The listing builds one solid part. Answer for the finished solid, in the listing's coordinates (mm). Face numbers are marked on the shaded views. A direction names the side the tool comes from. Round coordinates to 2 decimals unless told otherwise and drop trailing zeros. Write each loop counter-clockwise with the first axis right and the second up, starting at its lowest first coordinate (ties: lowest second). Pieces come first, ordered by that corner, then holes. Notation, with made-up numbers: M -0.5,37 L 16.5,37 A21 cw 16.5,52 Z; hole C 29.5,-30.5 d10. An arc over 180 degrees is marked long. Answer as CSV lines item,"result". Start each with the question number.
from build123d import *

# Parameters (mm, degrees)
SKETCH1_R           = 2.75
BOSS_EXTRUDE1_DEPTH = 6
BODY_START          = 3
SKETCH2_R           = 2.75
BODY_HOLE_DEPTH     = 3
CUT_EXTRUDE2_DEPTH  = 23.226110771
CUT_REVOLVE1_ANGLE  = 180
SKETCH7_R           = 0.8
SCREW_HOLES_DEPTH   = 22.656407828
SKETCH9_R           = 1.25
SCREW_HEADS_DEPTH   = 4


with BuildPart() as part:
    # Sketch1 → Boss-Extrude1 (new body)
    with BuildSketch(Plane.XY):
        with BuildLine():
            Line((17, -12), (17, 12))
            Line((17, 12), (5, 12))
            ThreePointArc((5, 12), (-13, 0), (5, -12))
            Line((5, -12), (17, -12))
        make_face()
        Circle(SKETCH1_R, mode=Mode.SUBTRACT)
    extrude(amount=BOSS_EXTRUDE1_DEPTH)

    # Sketch2 → Body Hole (cut)
    with BuildSketch(Plane.XY.offset(BODY_START)):
        with BuildLine():
            ThreePointArc((5, 12), (-13, 0), (5, -12))
            Line((5, -12), (13, -12))
            Line((13, -12), (13, -4.25))
            Line((13, -4.25), (17, -4.25))
            Line((17, -4.25), (17, 4.25))
            Line((17, 4.25), (13, 4.25))
            Line((13, 4.25), (13, 12))
            Line((13, 12), (5, 12))
        make_face()
        Circle(SKETCH2_R, mode=Mode.SUBTRACT)
    extrude(amount=BODY_HOLE_DEPTH, mode=Mode.SUBTRACT)

    # Sketch3 → Cut-Extrude2 (cut, through all)
    with BuildSketch(Plane(origin=(0, 0, 0), x_dir=(0, 0, -1), z_dir=(1, 0, 0))):
        with BuildLine():
            Line((2, 15), (-13, 15))
            ThreePointArc((-13, 15), (-2.393398282, 10.606601718), (2, 0))
            Line((2, 0), (2, 15))
        make_face()
        with BuildLine():
            Line((2, -15), (2, 0))
            ThreePointArc((2, 0), (-2.393398282, -10.606601718), (-13, -15))
            Line((-13, -15), (2, -15))
        make_face()
    extrude(amount=CUT_EXTRUDE2_DEPTH, mode=Mode.SUBTRACT)

    # Sketch6 → Cut-Revolve1 (revolve, cut)
    with BuildSketch(Plane(origin=(0, 0, 0), x_dir=(0, 0, -1), z_dir=(1, 0, 0))):
        with BuildLine():
            Line((1, 15), (-13, 15))
            ThreePointArc((-13, 15), (-4.508164866, 12.36481848), (1, 5.385164807))
            Line((1, 5.385164807), (2, 5.385164807))
            Line((2, 5.385164807), (2, 15))
            Line((2, 15), (1, 15))
        make_face()
    revolve(axis=Axis((0, 0, 0), (0, 0, 1)), revolution_arc=CUT_REVOLVE1_ANGLE, mode=Mode.SUBTRACT)

    # Sketch7 → Screw Holes (cut, through all)
    with BuildSketch(Plane.XY):
        with Locations(Location((15, 10, 0), (0, 0, 180))):
            Circle(SKETCH7_R)
        with Locations(Location((15, -10, 0), (0, 0, 180))):
            Circle(SKETCH7_R)
    extrude(amount=SCREW_HOLES_DEPTH, mode=Mode.SUBTRACT)

    # Sketch9 → Screw Heads (cut)
    with BuildSketch(Plane.XY):
        with Locations(Location((15, 10, 0), (0, 0, 180))):
            Circle(SKETCH9_R)
    extrude(amount=SCREW_HEADS_DEPTH, mode=Mode.SUBTRACT)


solid = part.part
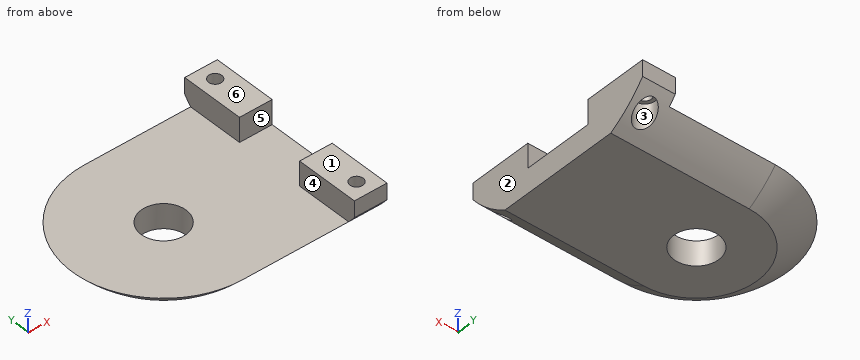
Q1. For the marked faces 4, 5 and 6, determine the directions among +Z, -Z, +X, -X, +Y, -Y from which every point of the face is accessible in a straight line to the end or side of a thin tool.
Q2. Straight lines are drawn through the part: L1, parallel to Y at x = 15, z = 5.05; L2, parallel to X at y = -10, z = 4.8; L3, parallel to Z at x = 14.5, y = 2. For each, find the intervals that lie inside material, in ascending order.
Q3. Find section B-B (y = 0). Determine the outline of the cut face in (x, z), plus the area to 3 significant figures.
Q4. Find section D-D (x = -2). Determine the outline of the cut face in (y, z).
Q5. Each of these flat-tipped pins is pushed along its axis until it touches: P1, Ø4, axis at x = -8, y = -2, coming from the +Z side; P2, Ø3, axis at x = 15, y = 10.5, coming from the -Z side; P3, Ø3.5, axis at x = 0, y = 0, coming from the -Z side; P4, Ø2, axis at y = 7, z = 1.5, coming from the -X side. Where does it stop, or does it pass through?
Q6. The mould has two halves that part along X. Classify the marked faces 1, 2 and 3: +X half, -X half, draft (parallel to the pull), parting line (faces both ways), or undercut.
Q7. Find section A-A (z = 5.25). Determine the outline of the cut face in (x, y).
Q8. Find section C-C (x = 15). Determine the outline of the cut face in (y, z), plus the area to 3 significant figures.
Reported:
1,face 4,"+Z, -X, +Y, -Y"
1,face 5,"+Z, +X, -X"
1,face 6,"+Z, +X, -X, +Y, -Y"
2,L1,"y = -12 to -10.8, -9.2 to -4.25, 4.25 to 9.2, 10.8 to 12"
2,L2,"x = 13 to 14.2, 15.8 to 17"
2,L3,"z = 0 to 3"
3,outline,"M -11.18,3 A15 ccw -7.48,0 L -2.75,0 L -2.75,3 Z; M 2.75,0 L 17,0 L 17,3 L 2.75,3 Z"
3,area,"63.1 mm2"
4,outline,"M -11,3 A14.87 ccw -7.21,0 L -1.89,0 L -1.89,3 Z; M 1.89,0 L 7.21,0 A14.87 ccw 11,3 L 1.89,3 Z"
5,P1,"stops at z = 3"
5,P2,"stops at z = 1.44"
5,P3,"passes through"
5,P4,"stops at x = -8.35"
6,face 1,"draft"
6,face 2,"+X half"
6,face 3,"undercut"
7,outline,"M 13,-12 L 17,-12 L 17,-4.25 L 13,-4.25 Z; M 13,4.25 L 17,4.25 L 17,12 L 13,12 Z; hole C 15,-10 d1.6; hole C 15,10 d1.6"
8,outline,"M -12,4 A15 ccw -10.8,2.59 L -10.8,6 L -12,6 Z; M -9.2,1.15 A15 ccw -7.48,0 L 7.48,0 A15 ccw 8.75,0.82 L 8.75,4 L 9.2,4 L 9.2,6 L 4.25,6 L 4.25,3 L -4.25,3 L -4.25,6 L -9.2,6 Z; M 10.8,4 L 11.25,4 L 11.25,3.08 A15 ccw 12,4 L 12,6 L 10.8,6 Z"
8,area,"87.7 mm2"
